```python
from build123d import *

# Parameters (mm, degrees)
F0_R     = 6.35
F1_DEPTH = 12.7


with BuildPart() as f1:
    # F0 (on Top) → F1 (new body)
    with BuildSketch(Plane.XY):
        with BuildLine():
            ThreePointArc((76.2, 0), (79.919744, -8.980256), (88.9, -12.7))
            ThreePointArc((88.9, -12.7), (97.880256, -8.980256), (101.6, 0))
            Line((101.6, 0), (101.6, 12.7))
            Line((101.6, 12.7), (101.6, 50.8))
            Line((101.6, 50.8), (101.6, 63.5))
            ThreePointArc((101.6, 63.5), (97.880256, 72.480256), (88.9, 76.2))
            ThreePointArc((88.9, 76.2), (79.919744, 72.480256), (76.2, 63.5))
            Line((76.2, 63.5), (76.2, 50.8))
            Line((76.2, 50.8), (12.7, 50.8))
            Line((12.7, 50.8), (12.7, 63.5))
            ThreePointArc((12.7, 63.5), (8.980256, 72.480256), (0, 76.2))
            ThreePointArc((0, 76.2), (-8.980256, 72.480256), (-12.7, 63.5))
            Line((-12.7, 63.5), (-12.7, 50.8))
            Line((-12.7, 50.8), (-12.7, 38.1))
            Line((-12.7, 38.1), (0, 38.1))
            ThreePointArc((0, 38.1), (4.490128, 36.240128), (6.35, 31.75))
            ThreePointArc((6.35, 31.75), (4.490128, 27.259872), (0, 25.4))
            Line((0, 25.4), (-12.7, 25.4))
            Line((-12.7, 25.4), (-12.7, 12.7))
            Line((-12.7, 12.7), (-12.7, 0))
            ThreePointArc((-12.7, 0), (-8.980256, -8.980256), (0, -12.7))
            ThreePointArc((0, -12.7), (8.980256, -8.980256), (12.7, 0))
            Line((12.7, 0), (12.7, 12.7))
            Line((12.7, 12.7), (76.2, 12.7))
            Line((76.2, 12.7), (76.2, 0))
        make_face()
        Circle(F0_R, mode=Mode.SUBTRACT)
        with Locations((88.9, 0)):
            Circle(F0_R, mode=Mode.SUBTRACT)
        with Locations((0, 63.5)):
            Circle(F0_R, mode=Mode.SUBTRACT)
        with Locations((88.9, 63.5)):
            Circle(F0_R, mode=Mode.SUBTRACT)
    extrude(amount=F1_DEPTH)


solid = f1.part
```
CAD build for the part. Positions are in the model's coordinates, mm. A direction names the side the tool comes from. Coordinates: 2 decimals unless noted, no trailing zeros. Order: outer loops, then holes, each group sorted by start corner. A loop starts at its lowest first (then second) coordinate and runs counter-clockwise, first axis right, second up. Notation, with made-up numbers: (38, 80) -> (89, 80) arc R26 ccw to (89, 96) -> close; hole circle Ø10 at (52, 41). An arc over 180 degrees is marked (long way). Use one line per item in the form item = value. Start each with the question number.
1) Band-saw the part on C-C on x = 52.5. Give the cut face in (y, z).
2) Band-saw the part on A-A on z = 9.5. Give the cut face in (x, y), then the cut area to 3 significant figures.
3) Drop flat-ended pins along their axis: pin 1 (1.5 mm diameter, centred on y = -1.5, z = 9, fed in from +X); pin 2 (4 mm diameter, centred on x = 42.5, z = 3, fed in from -Y); pin 3 (4 mm diameter, centred on x = -7.5, z = 4, fed in from +Y). Give the stop position or say it passes through.
4) Pull direction Y, two halves, no side cores. Call faces 1 (the flat face through (44, 12.7, 6)), 2 (the cylindrical face through (-1.38, -6.2, 6.26)), 3 (the flat face through (-12.7, 13, 6)): +Y half, -Y half, draft (parallel to the pull), parting line (faces both ways), or undercut.
5) Band-saw the part on B-B on y = 61.5. Give the cut face in (x, z), then the cut area to 3 significant figures.
6) Drill centre lines: L1, parallel to Y at x = 88.9, z = 9; L2, parallel to Y at x = 86.5, z = 3.5; L3, parallel to Y at x = 0, z = 3. Where is each one in solid material? Low to high. Write a range as [from, to].
7) Tool access for faces 4 (the flat face through (-6, 38.1, 6)), 5 (the flat face through (12.7, 6, 6)), 6 (the cylindrical face through (82.556, 0.279, 6.261)), 7 (the flat face through (45, 50.8, 6)): list every direction of +Z, -Z, +X, -X, +Y, -Y with a clear straight run to the whole face (end or side of a thin tool).
Entries:
q1.outline = (12.7, 0) -> (50.8, 0) -> (50.8, 12.7) -> (12.7, 12.7) -> close
q2.outline = (-12.7, 0) arc R12.7 ccw to (12.7, 0) -> (12.7, 12.7) -> (76.2, 12.7) -> (76.2, 0) arc R12.7 ccw to (101.6, 0) -> (101.6, 63.5) arc R12.7 ccw to (76.2, 63.5) -> (76.2, 50.8) -> (12.7, 50.8) -> (12.7, 63.5) arc R12.7 ccw to (-12.7, 63.5) -> (-12.7, 38.1) -> (0, 38.1) arc R6.35 cw to (0, 25.4) -> (-12.7, 25.4) -> close; hole circle Ø12.7 at (0, 0); hole circle Ø12.7 at (0, 63.5); hole circle Ø12.7 at (88.9, 0); hole circle Ø12.7 at (88.9, 63.5)
q2.area = 5,930 mm2
q3.pin_1 = 101.58
q3.pin_2 = 12.7
q3.pin_3 = 74.95
q4.face_1 = -Y half
q4.face_2 = undercut
q4.face_3 = draft
q5.outline = (-12.7, 0) -> (-6.03, 0) -> (-6.03, 12.7) -> (-12.7, 12.7) -> close; (6.03, 0) -> (12.7, 0) -> (12.7, 12.7) -> (6.03, 12.7) -> close; (76.2, 0) -> (82.87, 0) -> (82.87, 12.7) -> (76.2, 12.7) -> close; (94.93, 0) -> (101.6, 0) -> (101.6, 12.7) -> (94.93, 12.7) -> close
q5.area = 339 mm2
q6.L1 = [-12.7, -6.35], [6.35, 57.15], [69.85, 76.2]
q6.L2 = [-12.47, -5.88], [5.88, 57.62], [69.38, 75.97]
q6.L3 = [-12.7, -6.35], [6.35, 25.4], [38.1, 57.15], [69.85, 76.2]
q7.face_4 = +Z, -Z, -X
q7.face_5 = +Z, -Z, -Y
q7.face_6 = +Z, -Z
q7.face_7 = +Z, -Z, +Y
